Geometry: final body of the model. Coordinates: model frame, mm. A direction names the side the tool comes from. Give positions to 0.01 mm unless a question says otherwise; leave off trailing zeros. Order: outer loops, then holes, each group sorted by start corner. A loop starts at its lowest first (then second) coordinate and runs counter-clockwise, first axis right, second up. Notation, with made-up numbers: (56, 58.25) -> (71, 58.25) arc R26 cw to (71, 97.25) -> close; hole circle Ø2 at (50.25, -19). An arc over 180 degrees is marked (long way). One line per item, written item: value. Start each with the question number.
Autodesk Inventor part; units mm, degrees
ref_plane "YZ Plane" through (0, 0, 0) normal (1, 0, 0) x (0, 1, 0)
ref_plane "XZ Plane" through (0, 0, 0) normal (0, 1, 0) x (-1, 0, 0)
ref_plane "XY Plane" through (0, 0, 0) normal (0, 0, 1) x (1, 0, 0)
sketch "Boceto1" plane through (0, 0, 0) normal (0, 0, 1) x (1, 0, 0)
  line L0 (-13.5, 50) -> (13.5, 50)
  line L1 (13.5, 50) -> (13.5, 0)
  line L2 (13.5, 0) -> (-13.5, 0)
  line L3 (-13.5, 0) -> (-13.5, 50)
  line L4 (0, 0) -> (0, 50) construction
  line L5 (0, 34.815) -> (8.5, 29.9075)
  line L6 (8.5, 29.9075) -> (8.5, 20.0925)
  line L7 (8.5, 20.0925) -> (0, 15.185)
  line L8 (0, 15.185) -> (-8.5, 20.0925)
  line L9 (-8.5, 20.0925) -> (-8.5, 29.9075)
  line L10 (-8.5, 29.9075) -> (0, 34.815)
  line L11 (-8.5, 29.9075) -> (-13.5, 29.9075) construction
  line L12 (8.5, 29.9075) -> (13.5, 29.9075) construction
  point P0 (0, 25)
  dimension "d20" = 17
  dimension "d21" = 5
  dimension "d22" = 27
  dimension "d23" = 50
extrude "Extrusión1" add sketch "Boceto1" along normal blind 6
sketch "Boceto2" plane through (0, 0, 0) normal (0, 0, -1) x (-1, 0, 0)
  line L0 (-8.5, 20.0925) -> (-8.5, 29.9075)
  line L1 (-8.5, 29.9075) -> (0, 34.815)
  line L2 (0, 34.815) -> (8.5, 29.9075)
  line L3 (8.5, 29.9075) -> (8.5, 20.0925)
  line L4 (8.5, 20.0925) -> (0, 15.185)
  line L5 (0, 15.185) -> (-8.5, 20.0925)
  line L6 (13.5, 50) -> (-13.5, 50)
  line L7 (-13.5, 50) -> (-13.5, 0)
  line L8 (-13.5, 0) -> (13.5, 0)
  line L9 (13.5, 0) -> (13.5, 50)
  point P0 (0, 0)
extrude "Extrusión2" add sketch "Boceto2" along normal blind 6 contours L0 L1 L2 L3 L4 L5 | L9 L8 L7 L6
sketch "Boceto3" plane through (0, 0, -6) normal (0, 0, -1) x (-1, 0, 0)
  line L0 (0, 0) -> (0, 50) construction
  line L1 (-13.5, 50) -> (13.5, 50)
  circle A0 centre (0, 25) radius 5.5
  dimension "d18" = 11
extrude "Extrusión3" cut sketch "Boceto3" against normal up to next
sketch "Boceto5" plane through (0, 0, 6) normal (0, 0, 1) x (1, 0, 0)
  line L0 (-13.5, 0) -> (-13.5, 50)
  line L1 (13.5, 50) -> (13.5, 0)
  line L2 (-13.5, 0) -> (13.5, 0)
  line L3 (13.5, 0) -> (13.5, 12)
  line L4 (13.5, 12) -> (-13.5, 12)
  line L5 (-13.5, 12) -> (-13.5, 0)
  line L6 (13.5, 50) -> (-13.5, 50)
  line L7 (-13.5, 50) -> (13.5, 50)
  line L8 (13.5, 50) -> (13.5, 38)
  line L9 (13.5, 38) -> (-13.5, 38)
  line L10 (-13.5, 38) -> (-13.5, 50)
  line L11 (-17.3027, 25) -> (12.0796, 25) construction
  line L12 (-8.5, 20.0925) -> (-8.5, 29.9075)
  point P0 (0, 0)
  point P1 (-8.5, 25)
  dimension "d24" = 12
extrude "Extrusión4" add sketch "Boceto5" along normal blind 115 contours L0 L4 L1 L2 | L0 L6 L1 L9
sketch "Boceto9" plane through (-13.5, 0, -6) normal (0, -1, 0) x (1, 0, 0)
  circle A0 centre (13.5, 110) radius 5
  line L0 (0, 127) -> (27, 127)
  line L1 (13.5, 110) -> (13.5, 115)
  line L2 (13.5, 115) -> (13.5, 127)
  line L3 (0, 127) -> (27, 127)
  point P0 (13.5, 6)
  dimension "d25" = 10
  dimension "d32" = 12
extrude "Extrusión8" cut sketch "Boceto9" against normal up to surface (12 mm away)
sketch "Boceto10" plane through (0, 0, -6) normal (0, 0, -1) x (-1, 0, 0)
  circle A0 centre (0, 25) radius 11
  circle A1 centre (0, 25) radius 5.5
  point P0 (0, 0)
  dimension "d29" = 22
extrude "Extrusión9" cut sketch "Boceto10" against normal blind 2.5
sketch "Boceto11" plane through (-13.5, 12, 6) normal (0, 1, 0) x (1, 0, 0)
  line L0 (21.5, -106) -> (5.5, -106) construction
  line L1 (5.5, -106) -> (5.5, -90) construction
  line L2 (5.5, -90) -> (21.5, -90) construction
  line L3 (21.5, -90) -> (21.5, -106) construction
  line L4 (5.5, -106) -> (21.5, -90) construction
  circle A0 centre (13.5, -98) radius 8 construction
  circle A1 centre (13.5, -98) radius 11.3137
  line L5 (27, 0) -> (27, -115)
  circle A2 centre (13.5, -98) radius 5
  point P0 (13.5, 6)
  dimension "d45" = 16
extrude "Extrusión10" cut sketch "Boceto11" against normal blind 3 contours A1 | A2
sketch "Boceto12" plane through (-13.5, 0, -6) normal (0, -1, 0) x (1, 0, 0)
  circle A0 centre (13.5, 110) radius 11.3137
  line L0 (0, 127) -> (0, 0)
  point P0 (13.5, 6)
extrude "Extrusión11" cut sketch "Boceto12" against normal blind 3
sketch "Boceto14" plane through (-13.5, 50, -6) normal (0, 1, 0) x (1, 0, 0)
  circle A0 centre (13.5, -110) radius 5
  circle A1 centre (13.5, -110) radius 4
  point P0 (13.5, -6)
  dimension "d38" = 8
extrude "Extrusión12" cut sketch "Boceto14" against normal up to next contours A1
sketch "Boceto15" plane through (-13.5, 38, 6) normal (0, -1, 0) x (1, 0, 0)
  circle A0 centre (13.5, 98) radius 4
  circle A1 centre (13.5, 98) radius 8.25
  point P0 (13.5, -6)
  dimension "d41" = 16.5
extrude "Extrusión13" cut sketch "Boceto15" against normal blind 8
fillet "Empalme4" radius 12 4 edges at (13.5, 44, 121) (-13.5, 44, 121) (13.5, 6, 121) (-13.5, 6, 121)
fillet "Empalme5" radius 12 2 edges at (0, 0, -6) (0, 50, -6)
fillet "Empalme6" radius 12 2 edges at (0, 12, 6) (0, 38, 6)
properties part number "U3"
1. Cut plane A-A, the plane z = 46. Return loops of the section in (x, y), then the cut area to 3 significant figures.
2. Cut plane D-D, the plane z = 4. Return loops of the section in (x, y) (1 decimal), then the cut area to 3 significant figures.
3. Cut plane C-C, the plane y = 17. Return loops of the section in (x, z), then the cut area to 3 significant figures.
4. Draft query along Z for faces 1 (the cylindrical face through (-0.19, 3.61, -2.58)), 2 (the flat face through (0, 50, 63)), 3 (the cylindrical face through (-10.08, 6.08, 117.39)), 4 (the cylindrical face through (-2.453, 10.521, 115.045)). Return one class per face: pulls with the +Z half, pulls with the -Z half, needs draft (parallel to the pull), parting line crosses it, or undercut.
5. Cut plane B-B, the plane z = 104. Return loops of the section in (x, y), then the cut area to 3 significant figures.
6. Material intervals for L1, parallel to Y at x = -0.5, z = 55.5; L2, parallel to Y at x = -6.25, z = 95; L3, parallel to X at y = 9.9, z = 104, sorted ascending. Write a range as [from, to].
7. Access query for faces 5 (the flat face through (4.31, 17.673, 3.765)), 6 (the flat face through (5, 28, -3.5)), 7 (the cylindrical face through (-2.453, 1.479, 92.955)), 8 (the cylindrical face through (0.19, 46.39, -2.58)), 9 (the flat face through (0, 12, 57)). Directions: +Z, -Z, +X, -X, +Y, -Y. A direction counts if a zero-diameter tool reaches every point of the face in a straight line with its end or side. Return the directions, or none.
8. Pin query (flat end, axial travel): P1, Ø14.5, axis at x = 0, y = 25, coming from the -Z side; P2, Ø0.6, axis at x = 10.5, y = 25, coming from the +Z side; P3, Ø13, axis at x = 0, z = 104, coming from the -Y side. Return the tip coordinate at first contact, or that it passes through.
Answers follow:
1. outline: (-13.5, 0) -> (13.5, 0) -> (13.5, 12) -> (-13.5, 12) -> close; (-13.5, 38) -> (13.5, 38) -> (13.5, 50) -> (-13.5, 50) -> close
1. area: 648 mm²
2. outline: (-13.5, 0.2) -> (13.5, 0.2) -> (13.5, 49.8) -> (-13.5, 49.8) -> close; hole (-8.5, 20.1) -> (0, 15.2) -> (8.5, 20.1) -> (8.5, 29.9) -> (0, 34.8) -> (-8.5, 29.9) -> close
2. area: 1,090 mm²
3. outline: (-13.5, -6) -> (-7.55, -6) -> (-7.55, -3.5) -> (7.55, -3.5) -> (7.55, -6) -> (13.5, -6) -> (13.5, 8.25) -> (3.14, 8.25) -> (3.14, 0) -> (-3.14, 0) -> (-3.14, 8.25) -> (-13.5, 8.25) -> close
3. area: 295 mm²
4. face 1: pulls with the -Z half
4. face 2: needs draft
4. face 3: pulls with the +Z half
4. face 4: undercut
5. outline: (-13.5, 0) -> (-11.31, 0) -> (-11.31, 3) -> (-5, 3) -> (-5, 9) -> (-11.31, 9) -> (-11.31, 12) -> (-13.5, 12) -> close; (-13.5, 38) -> (-8.25, 38) -> (-8.25, 46) -> (-4, 46) -> (-4, 50) -> (-13.5, 50) -> close; (4, 46) -> (8.25, 46) -> (8.25, 38) -> (13.5, 38) -> (13.5, 50) -> (4, 50) -> close; (5, 3) -> (11.31, 3) -> (11.31, 0) -> (13.5, 0) -> (13.5, 12) -> (11.31, 12) -> (11.31, 9) -> (5, 9) -> close
5. area: 288 mm²
6. L1: y = [0, 12], [38, 50]
6. L2: y = [3, 9], [38, 50]
6. L3: x = [-13.5, -11.31], [11.31, 13.5]
7. face 5: +Z
7. face 6: -Z
7. face 7: -Y
7. face 8: -Z, +X, -X, +Y
7. face 9: +Z, +X, -X
8. P1: stops at z = -3.5
8. P2: stops at z = 6
8. P3: stops at y = 3
